```python
from build123d import *

# Parameters (mm, degrees)
BOSS_EXTRUDE1_DEPTH        = 10.668
SKETCH3_R                  = 2.54
CUT_EXTRUDE1_DEPTH         = 45.123624398
CHAMFER1_SIZE              = 0.00254
SKETCH4_W                  = 29.464
SKETCH4_H                  = 11.43
BOSS_EXTRUDE2_DEPTH        = 47.603865979
RIB1_REACH                 = 51.045
SKETCH5_WALL_W             = 117.009615236
SKETCH5_WALL_H             = 1.778
RIB2_REACH                 = 65.411
SKETCH6_WALL_W             = 145.742114112
SKETCH6_WALL_H             = 1.778
RIB3_START                 = -1.778
RIB3_DEPTH                 = 1.778
RIB4_START                 = -5.08
RIB4_DEPTH                 = 5.08
SKETCH9_W                  = 3.048
SKETCH9_H                  = 8.89
CUT_EXTRUDE2_DEPTH         = 60.891794651
SKETCH13_W                 = 2.54
SKETCH13_H                 = 8.128
BOSS_EXTRUDE3_DEPTH        = 0.254
SKETCH14_W                 = 0.762
SKETCH14_H                 = 0.762
CUT_EXTRUDE4_DEPTH         = 6.096
CHAMFER2_SIZE              = 0.508
LPATTERN1_COUNT            = 3
LPATTERN1_PITCH            = 2.54
CHAMFER2_OF_LPATTERN1_SIZE = 0.508
SKETCH15_W                 = 5.08
SKETCH15_H                 = 8.128
BOSS_EXTRUDE4_DEPTH        = 2.794
SKETCH16_W                 = 0.762
SKETCH16_H                 = 0.762
CUT_EXTRUDE5_DEPTH         = 6.096
CHAMFER3_SIZE              = 0.508
LPATTERN2_COUNT            = 3
LPATTERN2_PITCH            = 2.413
LPATTERN2_COUNT_DIR2       = 2
LPATTERN2_PITCH_DIR2       = 2.286
CHAMFER3_OF_LPATTERN2_SIZE = 0.508
SKETCH18_W                 = 8.382
SKETCH18_H                 = 8.382
CUT_EXTRUDE6_DEPTH         = 0.254
SKETCH19_R                 = 2.032
CUT_EXTRUDE7_DEPTH         = 45.380219265
MIRROR5_COPY_1_SKETCH_W    = 8.382
MIRROR5_COPY_1_SKETCH_H    = 8.382
MIRROR5_COPY_1_DEPTH       = 0.254
MIRROR5_COPY_2_SKETCH_R    = 2.032
MIRROR5_COPY_2_DEPTH       = 45.380219265


# Read off the part's stored shape, not the designer's step: Rib3, Rib4
with BuildPart() as part:
    # Sketch1 → Boss-Extrude1 (new body)
    with BuildSketch(Plane(origin=(0, 0, 0), x_dir=(1, 0, 0), z_dir=(0, 1, 0))):
        Polygon((0, 31.496), (7.239, 31.496), (14.553894525, 35.588705961), (20.903894525, 35.588705961), (23.801932989, 33.528), (23.801932989, 0), (0, 0), align=None)
    boss_extrude1 = extrude(amount=BOSS_EXTRUDE1_DEPTH)

    # Sketch3 → Cut-Extrude1 (cut, through all)
    with BuildSketch(Plane(origin=(0, 10.668, 0), x_dir=(1, 0, 0), z_dir=(0, 1, 0))):
        with Locations(Location((19.483932989, 31.524705961, 0), (0, 0, 270))):
            Circle(SKETCH3_R)
    cut_extrude1 = extrude(amount=-CUT_EXTRUDE1_DEPTH, mode=Mode.SUBTRACT)

    # Mirror1: Boss-Extrude1, Cut-Extrude1 across plane
    add(boss_extrude1.mirror(Plane(origin=(0, 0, 0), x_dir=(0, 0, 1), z_dir=(1, 0, 0))))
    add(cut_extrude1.mirror(Plane(origin=(0, 0, 0), x_dir=(0, 0, 1), z_dir=(1, 0, 0))), mode=Mode.SUBTRACT)

    # Mirror2: part across plane


with BuildPart() as part_1:
    add(part.part)
    add(part.part.mirror(Plane.XY))

    # Chamfer1
    chamfer1_edges = [part_1.edges().sort_by_distance(p)[0] for p in [
        (0, 10.668, -31.496),
        (0, 10.668, 31.496),
    ]]
    chamfer(chamfer1_edges, length=CHAMFER1_SIZE)

    # Sketch4 → Boss-Extrude2 (add)
    with BuildSketch(Plane(origin=(23.801932989, 0, 0), x_dir=(0, 0, -1), z_dir=(1, 0, 0))):
        with Locations((0, 16.383)):
            Rectangle(SKETCH4_W, SKETCH4_H)
    extrude(amount=-BOSS_EXTRUDE2_DEPTH)

    # Sketch5 wall → Rib1 (add, up to next)
    with BuildSketch(Plane(origin=(-1.703932989, 16.383, 20.96935298), x_dir=(0, -0.675559301544, 0.737305655816), z_dir=(0, -0.737305655816, -0.675559301544)), mode=Mode.PRIVATE) as rib1_sk1:
        with Locations((0, -0.889)):
            Rectangle(SKETCH5_WALL_W, SKETCH5_WALL_H)
    rib1_tool1 = extrude(rib1_sk1.sketch, amount=RIB1_REACH, mode=Mode.PRIVATE) - part_1.part
    rib1 = rib1_tool1.solids().sort_by_distance((-1.703932989, 16.383, 20.96935298))[0]
    add(rib1)

    # Sketch6 wall → Rib2 (add, up to next)
    with BuildSketch(Plane(origin=(23.801932989, 16.383, 20.96935298), x_dir=(0, -0.675559301544, 0.737305655816), z_dir=(0, -0.737305655816, -0.675559301544)), mode=Mode.PRIVATE) as rib2_sk1:
        with Locations((0, 0.889)):
            Rectangle(SKETCH6_WALL_W, SKETCH6_WALL_H)
    rib2_tool1 = extrude(rib2_sk1.sketch, amount=RIB2_REACH, mode=Mode.PRIVATE) - part_1.part
    rib2 = rib2_tool1.solids().sort_by_distance((23.801932989, 16.383, 20.96935298))[0]
    add(rib2)

    # Rib3 outline → Rib3 (add)
    with BuildSketch(Plane.ZY.offset(23.801932989).offset(RIB3_START)):
        Polygon((27.206705961, 10.668), (14.732, 22.098), (14.732, 10.668), align=None)
    rib3 = extrude(amount=RIB3_DEPTH)

    # Rib4 outline → Rib4 (add)
    with BuildSketch(Plane.ZY.offset(-12.012067011).offset(RIB4_START)):
        Polygon((27.206705961, 10.668), (14.732, 22.098), (14.732, 10.668), align=None)
    extrude(amount=RIB4_DEPTH)

    # Sketch9 → Cut-Extrude2 (cut, through all)
    with BuildSketch(Plane.XY.offset(14.732)):
        with Locations((14.552067011, 17.653)):
            Rectangle(SKETCH9_W, SKETCH9_H)
    extrude(amount=CUT_EXTRUDE2_DEPTH, mode=Mode.SUBTRACT)

    # Sketch13 → Boss-Extrude3 (add)
    with BuildSketch(Plane(origin=(0, 13.208, 0), x_dir=(1, 0, 0), z_dir=(0, 1, 0))):
        with Locations((14.552067011, -19.583274541)):
            Rectangle(SKETCH13_W, SKETCH13_H)
    extrude(amount=BOSS_EXTRUDE3_DEPTH)

    # Sketch14 → Cut-Extrude4 (cut)
    with BuildSketch(Plane(origin=(0, 13.462, 0), x_dir=(1, 0, 0), z_dir=(0, 1, 0))):
        with Locations((14.552067011, -17.043274541)):
            Rectangle(SKETCH14_W, SKETCH14_H)
    cut_extrude4 = extrude(amount=-CUT_EXTRUDE4_DEPTH, mode=Mode.SUBTRACT)

    # Chamfer2
    chamfer2_edges = [part_1.edges().sort_by_distance(p)[0] for p in [
        (14.933067011, 13.462, 17.043274541),
        (14.552067011, 13.462, 16.662274541),
        (14.171067011, 13.462, 17.043274541),
        (14.552067011, 13.462, 17.424274541),
    ]]
    chamfer(chamfer2_edges, length=CHAMFER2_SIZE)

    # LPattern1: Cut-Extrude4 ×3
    with Locations(*[(0, 0, i * LPATTERN1_PITCH) for i in range(1, LPATTERN1_COUNT)]):
        add(cut_extrude4, mode=Mode.SUBTRACT)

    # Chamfer2 of LPattern1
    chamfer2_of_lpattern1_edges = [part_1.edges().sort_by_distance(p)[0] for p in [
        (14.933067011, 13.462, 19.583274541),
        (14.552067011, 13.462, 19.202274541),
        (14.171067011, 13.462, 19.583274541),
        (14.552067011, 13.462, 19.964274541),
        (14.933067011, 13.462, 22.123274541),
        (14.552067011, 13.462, 21.742274541),
        (14.171067011, 13.462, 22.123274541),
        (14.552067011, 13.462, 22.504274541),
    ]]
    chamfer(chamfer2_of_lpattern1_edges, length=CHAMFER2_OF_LPATTERN1_SIZE)

    # Mirror3: Rib1, Rib2, Rib3 across plane
    add(rib1.mirror(Plane.XY))
    add(rib2.mirror(Plane.XY))
    add(rib3.mirror(Plane.XY))

    # Sketch15 → Boss-Extrude4 (add)
    with BuildSketch(Plane(origin=(0, 10.668, 0), x_dir=(1, 0, 0), z_dir=(0, 1, 0))):
        with Locations((17.197932989, 20.32)):
            Rectangle(SKETCH15_W, SKETCH15_H)
    extrude(amount=BOSS_EXTRUDE4_DEPTH)

    # Sketch16 → Cut-Extrude5 (cut)
    with BuildSketch(Plane(origin=(0, 13.462, 0), x_dir=(1, 0, 0), z_dir=(0, 1, 0))):
        with Locations((18.340932989, 17.907)):
            Rectangle(SKETCH16_W, SKETCH16_H)
    cut_extrude5 = extrude(amount=-CUT_EXTRUDE5_DEPTH, mode=Mode.SUBTRACT)

    # Chamfer3
    chamfer3_edges = [part_1.edges().sort_by_distance(p)[0] for p in [
        (18.721932989, 13.462, -17.907),
        (18.340932989, 13.462, -18.288),
        (17.959932989, 13.462, -17.907),
        (18.340932989, 13.462, -17.526),
    ]]
    chamfer(chamfer3_edges, length=CHAMFER3_SIZE)

    # LPattern2: Cut-Extrude5 3 × 2
    with Locations(*[(-j * LPATTERN2_PITCH_DIR2, 0, -i * LPATTERN2_PITCH) for i in range(LPATTERN2_COUNT) for j in range(LPATTERN2_COUNT_DIR2) if (i, j) != (0, 0)]):
        add(cut_extrude5, mode=Mode.SUBTRACT)

    # Chamfer3 of LPattern2
    chamfer3_of_lpattern2_edges = [part_1.edges().sort_by_distance(p)[0] for p in [
        (16.435932989, 13.462, -17.907),
        (16.054932989, 13.462, -18.288),
        (15.673932989, 13.462, -17.907),
        (16.054932989, 13.462, -17.526),
        (18.721932989, 13.462, -20.32),
        (18.340932989, 13.462, -20.701),
        (17.959932989, 13.462, -20.32),
        (18.340932989, 13.462, -19.939),
        (16.435932989, 13.462, -20.32),
        (16.054932989, 13.462, -20.701),
        (15.673932989, 13.462, -20.32),
        (16.054932989, 13.462, -19.939),
        (18.721932989, 13.462, -22.733),
        (18.340932989, 13.462, -23.114),
        (17.959932989, 13.462, -22.733),
        (18.340932989, 13.462, -22.352),
        (16.435932989, 13.462, -22.733),
        (16.054932989, 13.462, -23.114),
        (15.673932989, 13.462, -22.733),
        (16.054932989, 13.462, -22.352),
    ]]
    chamfer(chamfer3_of_lpattern2_edges, length=CHAMFER3_OF_LPATTERN2_SIZE)

    # Sketch18 → Cut-Extrude6 (cut)
    with BuildSketch(Plane(origin=(0, 10.668, 0), x_dir=(1, 0, 0), z_dir=(0, 1, 0))):
        with Locations((6.297067011, -20.193)):
            Rectangle(SKETCH18_W, SKETCH18_H)
    cut_extrude6 = extrude(amount=-CUT_EXTRUDE6_DEPTH, mode=Mode.SUBTRACT)

    # Sketch19 → Cut-Extrude7 (cut, through all)
    with BuildSketch(Plane(origin=(0, 10.414, 0), x_dir=(1, 0, 0), z_dir=(0, 1, 0))):
        with Locations(Location((6.297067011, -20.193, 0), (0, 0, 270))):
            Circle(SKETCH19_R)
    cut_extrude7 = extrude(amount=-CUT_EXTRUDE7_DEPTH, mode=Mode.SUBTRACT)

    # Mirror4: Cut-Extrude6, Cut-Extrude7 across plane
    add(cut_extrude6.mirror(Plane.ZY.offset(0.814932989)), mode=Mode.SUBTRACT)
    add(cut_extrude7.mirror(Plane.ZY.offset(0.814932989)), mode=Mode.SUBTRACT)

    # Mirror5: Cut-Extrude6, Cut-Extrude7 across plane
    add(cut_extrude6.mirror(Plane.XY), mode=Mode.SUBTRACT)
    add(cut_extrude7.mirror(Plane.XY), mode=Mode.SUBTRACT)

    # Mirror5 copy 1 sketch → Mirror5 copy 1 (cut)
    with BuildSketch(Plane(origin=(-1.629865979, 10.668, 0), x_dir=(-1, 0, 0), z_dir=(0, 1, 0))):
        with Locations((6.297067011, -20.193)):
            Rectangle(MIRROR5_COPY_1_SKETCH_W, MIRROR5_COPY_1_SKETCH_H)
    extrude(amount=-MIRROR5_COPY_1_DEPTH, mode=Mode.SUBTRACT)

    # Mirror5 copy 2 sketch → Mirror5 copy 2 (cut, through all)
    with BuildSketch(Plane(origin=(-1.629865979, 10.414, 0), x_dir=(-1, 0, 0), z_dir=(0, 1, 0))):
        with Locations(Location((6.297067011, -20.193, 0), (0, 0, 270))):
            Circle(MIRROR5_COPY_2_SKETCH_R)
    extrude(amount=-MIRROR5_COPY_2_DEPTH, mode=Mode.SUBTRACT)


solid = part_1.part
```
The listing builds one solid part. Answer for the finished solid, in the listing's coordinates (mm). A direction names the side the tool comes from. Coordinates: 2 decimals unless noted, no trailing zeros. Write each loop counter-clockwise with the first axis right and the second up, starting at its lowest first coordinate (ties: lowest second). Pieces come first, ordered by that corner, then holes. Notation, with made-up numbers: M 43,37.5 L 60,37.5 A22 cw 60,47.5 Z; hole C 87.25,28 d6. An arc over 180 degrees is marked long. Use a Markdown table: item, result. Add a question column.
1. For a pull along Z with two mould halves and no side action, classify faces 1 (the flat face through (10.84, 5.26, 33.51)), 2 (the cylindrical face through (21.626, 5.409, -30.159)), 3 (the flat face through (-23.802, 9, 0)) as +Z half, -Z half, draft (parallel to the pull), parting line (faces both ways), or undercut.
2. Section B-B (y = 17.5) is taken. Give the vertices of the cut face in (x, z).
3. Straight lines are drawn through the part: line 1 along X through (y, z) = (16, -15); line 2 along Z through (x, y) = (19, 10.75); line 3 along Z through (x, y) = (-20, 19.75). For each, find the intervals that lie inside material, in ascending order. Write a range as [from, to].
4. Which of the six approach directions +Z, -Z, +X, -X, +Y, -Y give full straight-line access (tool end or side, diameter ignored) to faces 4 (the flat face through (-1.704, 14, 19)), 5 (the flat face through (-12, 16, -14.732)), 6 (the flat face through (-7, 10.414, -18)), 7 (the flat face through (-10.84, 5.26, 33.51))?
5. Given P1, Ø4, axis at x = 7.5, z = -21, coming from the +Y side; P2, Ø1, axis at x = 12, y = 10.5, coming from the -Z side; P3, Ø0.6, axis at x = 14.5, z = 20, coming from the +Y side, each flat-ended and moving along its own axis, determine where each tip first touches the part or whether it passes through.
Data:
| question | item | result |
|---|---|---|
| 1 | face 1 | +Z half |
| 1 | face 2 | undercut |
| 1 | face 3 | draft |
| 2 | outline | M -23.8,-19.75 L -22.02,-19.75 L -22.02,-14.73 L -1.7,-14.73 L -1.7,-19.75 L 0.07,-19.75 L 0.07,-14.73 L 22.02,-14.73 L 22.02,-19.75 L 23.8,-19.75 L 23.8,19.75 L 22.02,19.75 L 22.02,14.73 L 17.09,14.73 L 17.09,19.75 L 16.08,19.75 L 16.08,14.73 L 13.03,14.73 L 13.03,19.75 L 12.01,19.75 L 12.01,14.73 L 0.07,14.73 L 0.07,19.75 L -1.7,19.75 L -1.7,14.73 L -22.02,14.73 L -22.02,19.75 L -23.8,19.75 Z |
| 3 | line 1 | x = [-23.8, -22.02], [-1.7, 0.07], [22.02, 23.8] |
| 3 | line 2 | z = [-24.38, -16.26], [-14.73, 14.73] |
| 3 | line 3 | z = [-14.73, 14.73] |
| 4 | face 4 | +Z, +Y |
| 4 | face 5 | -Z, +Y |
| 4 | face 6 | +Y |
| 4 | face 7 | +Z, +Y, -Y |
| 5 | P1 | stops at y = 10.41 |
| 5 | P2 | stops at z = -34.44 |
| 5 | P3 | stops at y = 13.29 |
